Source: CAD feature listing. Evaluate the final solid. Frame: model axes, mm. A direction names the side the tool comes from. Give positions to 0.01 mm unless a question says otherwise; leave off trailing zeros. Write each loop counter-clockwise with the first axis right and the second up, starting at its lowest first coordinate (ties: lowest second). Pieces come first, ordered by that corner, then holes.
```python
from build123d import *

# Parameters (mm, degrees)
F0_R     = 21.4249
F0_R_2   = 15
F0_R_3   = 10
F1_DEPTH = 6
F0_R_4   = 25
F2_DEPTH = 12
F4_W     = 10
F4_H     = 6
F5_DEPTH = 25


with BuildPart() as f1:
    # F0 (on Top) → F1 (new body)
    with BuildSketch(Plane.XY):
        Circle(F0_R)
        Circle(F0_R_2, mode=Mode.SUBTRACT)
        Circle(F0_R_2)
        Circle(F0_R_3, mode=Mode.SUBTRACT)
    extrude(amount=-F1_DEPTH)

    # F0 (on Top) → F2 (join)
    with BuildSketch(Plane.XY):
        Circle(F0_R_4)
        Circle(F0_R, mode=Mode.SUBTRACT)
    extrude(amount=-F2_DEPTH)

    # F4 (on Top) → F5 (cut)
    with BuildSketch(Plane.XY):
        with Locations((25, 0)):
            Rectangle(F4_W, F4_H)
        with Locations((-25, 0)):
            Rectangle(F4_W, F4_H)
    extrude(amount=-F5_DEPTH, mode=Mode.SUBTRACT)


solid = f1.part
```
1. Cut plane B-B, the plane y = 0. Return the cut outline in (x, z), then the cut area to 3 significant figures.
2. Cut plane D-D, the plane z = -8.75. Return the cut outline in (x, y), then the cut area to 3 significant figures.
3. Line query: L1, parallel to Y at x = 0, z = -2.7; L2, parallel to Z at x = -3.5, y = -16.5; L3, parallel to Y at x = 17, z = -11. Output: solid intervals per line, ascending.
4. Access query for faces 1 (the cylindrical face through (0.43, 21.42, -8.96)), 2 (the cylindrical face through (-0.508, -24.995, -5.916)), 3 (the flat face through (22, -3, -6)), 4 (the flat face through (-22, -3, -6)). Directions: +Z, -Z, +X, -X, +Y, -Y. A direction counts if a zero-diameter tool reaches every point of the face in a straight line with its end or side. Return the directions, or none.
5. Cut plane A-A, the plane x = 0. Return the cut outline in (y, z).
6. Mould query, pull axis Y, two halves, no side actions, for faces 5 (the cylindrical face through (0.508, 24.995, -5.916)), 6 (the flat face through (11, 0, 0)), 7 (the flat face through (20, 0, -3)). Classes: +Y half, -Y half, draft (parallel to the pull), parting line (faces both ways), or undercut.
7. Cut plane C-C, the plane z = -1.75. Return the cut outline in (x, y), then the cut area to 3 significant figures.
8. Contact query for flat-ended pins moving along their axis: P1, Ø6, axis at x = -6, z = -8.5, coming from the -Y side; P2, Ø8, axis at x = -10.5, y = 11, coming from the -Z side; P3, Ø3, axis at y = 8.5, z = -1.5, coming from the -X side. Output: stop coordinate, or through.
Response values:
1. outline: (-20, -6) - (-10, -6) - (-10, 0) - (-20, 0) - close; (10, -6) - (20, -6) - (20, 0) - (10, 0) - close
1. area: 120 mm2
2. outline: (-24.82, -3) arc R25 ccw to (24.82, -3) - (21.21, -3) arc R21.42 cw to (-21.21, -3) - close; (-24.82, 3) - (-21.21, 3) arc R21.42 cw to (21.21, 3) - (24.82, 3) arc R25 ccw to start
2. area: 478 mm2
3. L1: y = -25 to -10, 10 to 25
3. L2: z = -6 to 0
3. L3: y = -18.33 to -13.04, 13.04 to 18.33
4. face 1: -Z
4. face 2: +Z, -Z, -Y
4. face 3: +Z, -Z, +X
4. face 4: +Z, -Z, -X
5. outline: (-25, -12) - (-21.42, -12) - (-21.42, -6) - (-10, -6) - (-10, 0) - (-25, 0) - close; (10, -6) - (21.42, -6) - (21.42, -12) - (25, -12) - (25, 0) - (10, 0) - close
6. face 5: +Y half
6. face 6: draft
6. face 7: undercut
7. outline: (-24.82, -3) arc R25 ccw to (24.82, -3) - (20, -3) - (20, 3) - (24.82, 3) arc R25 ccw to (-24.82, 3) - (-20, 3) - (-20, -3) - close; hole circle Ø20 at (0, 0)
7. area: 1,590 mm2
8. P1: stops at y = -24.82
8. P2: stops at z = -6
8. P3: stops at x = -24
